```python
from build123d import *

# Parameters (mm, degrees)
CYLINDER658_R               = 1.5
CYLINDER658_DEPTH           = 20
CYLINDER658_PLACEMENT_ANGLE = 45
CYLINDER659_R               = 1.5
CYLINDER659_DEPTH           = 20
CYLINDER652_R               = 1.5
CYLINDER652_DEPTH           = 20
CYLINDER652_PLACEMENT_ANGLE = 135
CYLINDER655_R               = 1.5
CYLINDER655_DEPTH           = 20
CYLINDER657_R               = 1.5
CYLINDER657_DEPTH           = 20
CYLINDER657_PLACEMENT_ANGLE = 225
CYLINDER654_R               = 1.5
CYLINDER654_DEPTH           = 20
CYLINDER656_R               = 1.5
CYLINDER656_DEPTH           = 20
CYLINDER656_PLACEMENT_ANGLE = 45
CYLINDER653_R               = 1.5
CYLINDER653_DEPTH           = 20
COMPOUND660_PLACEMENT_ANGLE = 22.5
TUBE040_R                   = 52
TUBE040_R_2                 = 42
TUBE040_DEPTH               = 3
CHAMFER018_SIZE             = 1


with BuildPart() as obj1:
    # Cylinder658 → Cylinder658 (new body)
    with BuildSketch(Plane.XY):
        Circle(CYLINDER658_R)
    extrude(amount=CYLINDER658_DEPTH)


with BuildPart() as obj1_1:
    # Cylinder658 placement: moved
    add(obj1.part.moved(Location((-31.819805, 31.819805, -18))).rotate(Axis((-31.819805, 31.819805, -18), (0, 0, 1)), CYLINDER658_PLACEMENT_ANGLE))


with BuildPart() as obj2:
    # Cylinder659 → Cylinder659 (new body)
    with BuildSketch(Plane(origin=(-45, 0, -18), x_dir=(0, 1, 0), z_dir=(0, 0, 1))):
        Circle(CYLINDER659_R)
    extrude(amount=CYLINDER659_DEPTH)


with BuildPart() as obj3:
    # Cylinder652 → Cylinder652 (new body)
    with BuildSketch(Plane.XY):
        Circle(CYLINDER652_R)
    extrude(amount=CYLINDER652_DEPTH)


with BuildPart() as obj3_1:
    # Cylinder652 placement: moved
    add(obj3.part.moved(Location((-31.819805, -31.819805, -18))).rotate(Axis((-31.819805, -31.819805, -18), (0, 0, 1)), CYLINDER652_PLACEMENT_ANGLE))


with BuildPart() as obj4:
    # Cylinder655 → Cylinder655 (new body)
    with BuildSketch(Plane(origin=(0, -45, -18), x_dir=(-1, 0, 0), z_dir=(0, 0, 1))):
        Circle(CYLINDER655_R)
    extrude(amount=CYLINDER655_DEPTH)


with BuildPart() as obj5:
    # Cylinder657 → Cylinder657 (new body)
    with BuildSketch(Plane.XY):
        Circle(CYLINDER657_R)
    extrude(amount=CYLINDER657_DEPTH)


with BuildPart() as obj5_1:
    # Cylinder657 placement: moved
    add(obj5.part.moved(Location((31.819805, -31.819805, -18))).rotate(Axis((31.819805, -31.819805, -18), (0, 0, 1)), CYLINDER657_PLACEMENT_ANGLE))


with BuildPart() as obj6:
    # Cylinder654 → Cylinder654 (new body)
    with BuildSketch(Plane(origin=(45, 0, -18), x_dir=(0, -1, 0), z_dir=(0, 0, 1))):
        Circle(CYLINDER654_R)
    extrude(amount=CYLINDER654_DEPTH)


with BuildPart() as obj7:
    # Cylinder656 → Cylinder656 (new body)
    with BuildSketch(Plane.XY):
        Circle(CYLINDER656_R)
    extrude(amount=CYLINDER656_DEPTH)


with BuildPart() as obj7_1:
    # Cylinder656 placement: moved
    add(obj7.part.moved(Location((31.819805, 31.819805, -18))).rotate(Axis((31.819805, 31.819805, -18), (0, 0, -1)), CYLINDER656_PLACEMENT_ANGLE))


with BuildPart() as compound660:
    # Cylinder653 → Cylinder653 (new body)
    with BuildSketch(Plane(origin=(0, 45, -18), x_dir=(1, 0, 0), z_dir=(0, 0, 1))):
        Circle(CYLINDER653_R)
    extrude(amount=CYLINDER653_DEPTH)

    # Compound660: union obj1, obj2, obj3, obj4, obj5, obj6, obj7
    add(obj1_1.part)
    add(obj2.part)
    add(obj3_1.part)
    add(obj4.part)
    add(obj5_1.part)
    add(obj6.part)
    add(obj7_1.part)


with BuildPart() as compound660_1:
    # Compound660 placement: moved
    add(compound660.part.rotate(Axis((0, 0, 0), (0, 0, 1)), COMPOUND660_PLACEMENT_ANGLE))


with BuildPart() as j_max_motor_high_washer_a:
    # Tube040 → Tube040 (new body)
    with BuildSketch(Plane.XY.offset(-11)):
        Circle(TUBE040_R)
        Circle(TUBE040_R_2, mode=Mode.SUBTRACT)
    extrude(amount=TUBE040_DEPTH)

    # Cut290: cut Compound660
    add(compound660_1.part, mode=Mode.SUBTRACT)


with BuildPart() as j_max_motor_high_washer_a_1:
    # Cut290 placement: moved
    add(j_max_motor_high_washer_a.part.moved(Location((0, 0, -4))))

    # Chamfer018
    chamfer018_edges = [j_max_motor_high_washer_a_1.edges().sort_by_distance(p)[0] for p in [
        (-52, 0, -15),
    ]]
    chamfer(chamfer018_edges, length=CHAMFER018_SIZE)


with BuildPart() as j_max_motor_high_washer_a_2:
    # Chamfer018 placement: moved
    add(j_max_motor_high_washer_a_1.part.moved(Location((0, 0, 4))))


solid = j_max_motor_high_washer_a_2.part
```
Can you work these out from the model? Positions are in its coordinate system, mm. Coordinates: 2 decimals unless noted, no trailing zeros. Loops run counter-clockwise (first coordinate to the right, second up) from the corner with the lowest first, then second, coordinate; pieces in that order, holes last.
1) For pin 1 (4 mm diameter, centred on x = 17.22, y = -41.57, fed in from +Z); pin 2 (1 mm diameter, centred on x = -2.5, z = -9.5, fed in from -Y), each with a flat end and sliding along its axis, tell me the tip position at first contact or that it passes through.
2) Thinking about a two-plate mould opening in X: for faces 1 (the cylindrical face through (-41.265, -31.641, -9.014)), 2 (the flat face through (4, 43, -8)), 3 (the cylindrical face through (40.097, 16.961, -9.521)), which applies, pulls with the +X half, pulls with the -X half, needs draft (parallel to the pull), parting line crosses it, or undercut?
3) Imagine slicing it at C-C on z = -10.5. State how many separate pieces and enclosed holes the cut face has, plus the area to 3 significant figures.
4) I need wall thicknesses on probe 1 along Y at (x, z) = (18.5, -10.35); probe 2 along Y at (x, z) = (0, -9.9); probe 3 along Y at (x, z) = (16.5, -8.85). Which ranges of each line are inside material? Lowest first, please.
5) Imagine slicing it at A-A on y = 0. List the corners of the cut face in (x, z) for me.
Completed:
1. pin 1: stops at z = -8
1. pin 2: stops at y = -51.96
2. face 1: parting line crosses it
2. face 2: needs draft
2. face 3: undercut
3. separate pieces: 1
3. enclosed holes: 9
3. area: 2,730 mm2
4. probe 1: y = -48.22 to -42.36, -40.79 to -37.71, 37.71 to 40.79, 42.36 to 48.22
4. probe 2: y = -52 to -42, 42 to 52
4. probe 3: y = -49.31 to -42.89, -40.26 to -38.62, 38.62 to 40.26, 42.89 to 49.31
5. outline: (-52, -10) - (-51, -11) - (-42, -11) - (-42, -8) - (-52, -8) - close; (42, -11) - (51, -11) - (52, -10) - (52, -8) - (42, -8) - close
